from build123d import *

# Parameters (mm, degrees)
BOSS_EXTRUDE1_DEPTH = 34.5
FILLET1_R           = 1
CUT_EXTRUDE1_DEPTH  = 8
FILLET2_R           = 5
SKETCH3_R           = 1.25
CUT_EXTRUDE2_DEPTH  = 8


with BuildPart() as part:
    # Sketch1 → Boss-Extrude1 (new body, symmetric)
    with BuildSketch(Plane.XY):
        with BuildLine():
            Line((-12, -1), (-2.987055406, -1))
            ThreePointArc((-2.987055406, -1), (0, -3.15), (2.987055406, -1))
            Line((2.987055406, -1), (12, -1))
            Line((12, -1), (12, -8))
            Line((12, -8), (-12, -8))
            Line((-12, -8), (-12, -1))
        make_face()
    extrude(amount=BOSS_EXTRUDE1_DEPTH, both=True)

    # Fillet1
    fillet1_edges = [part.edges().sort_by_distance(p)[0] for p in [
        (-2.987055406, -1, 0),
        (2.987055406, -1, 0),
    ]]
    fillet(fillet1_edges, radius=FILLET1_R)

    # Sketch2 → Cut-Extrude1 (cut, through all)
    with BuildSketch(Plane(origin=(0, -1, 0), x_dir=(1, 0, 0), z_dir=(0, 1, 0))):
        Polygon((-12, 27.5), (-5, 19.686646885), (-5, -19.686646885), (-12, -27.5), align=None)
        Polygon((12, -27.5), (5, -19.686646885), (5, 19.686646885), (12, 27.5), align=None)
    extrude(amount=-CUT_EXTRUDE1_DEPTH, mode=Mode.SUBTRACT)

    # Fillet2
    fillet2_edges = [part.edges().sort_by_distance(p)[0] for p in [
        (-12, -4.5, 27.5),
        (-12, -4.5, -27.5),
        (-5, -4.5, -19.686646885),
        (-5, -4.5, 19.686646885),
        (12, -4.5, -27.5),
        (12, -4.5, 27.5),
        (5, -4.5, 19.686646885),
        (5, -4.5, -19.686646885),
    ]]
    fillet(fillet2_edges, radius=FILLET2_R)

    # Sketch3 → Cut-Extrude2 (cut, through all)
    with BuildSketch(Plane(origin=(0, -1, 0), x_dir=(1, 0, 0), z_dir=(0, 1, 0))):
        with Locations((5.25, 29.610191819)):
            Circle(SKETCH3_R)
        with Locations((-5.25, 29.610191819)):
            Circle(SKETCH3_R)
        with Locations((-5.25, -29.610191819)):
            Circle(SKETCH3_R)
        with Locations((5.25, -29.610191819)):
            Circle(SKETCH3_R)
    extrude(amount=-CUT_EXTRUDE2_DEPTH, mode=Mode.SUBTRACT)


solid = part.part
Design review of the part built by this model. Coordinates are the model's own, in mm. A direction names the side the tool comes from. Coordinates: 2 decimals unless noted, no trailing zeros. Order: outer loops, then holes, each group sorted by start corner. A loop starts at its lowest first (then second) coordinate and runs counter-clockwise, first axis right, second up. Notation, with made-up numbers: (60, 84) -> (92, 84) arc R20 cw to (92, 105) -> close; hole circle Ø8 at (-25.5, 22.5). An arc over 180 degrees is marked (long way). One line per item, written item: value.
1) Draft analysis for pull direction X (two halves, no side actions). For faces 4 (the face through (4.98, -4.45, -28.39)), 5 (the face through (-11.66, -4.55, 27.6)), 6 (the face through (5.32, -4.55, 19.54)), state which applies: +X half, -X half, draft (parallel to the pull), parting line (faces both ways), or undercut.
Output values:
face 4: undercut
face 5: -X half
face 6: +X half
2) We need section A-A, the plane z = 8. Give the boundary of the cut face in (x, y).
Output values:
outline: (-5, -8) -> (5, -8) -> (5, -1) -> (3.64, -1) arc R1 ccw to (2.76, -1.52) arc R3.15 cw to (-2.76, -1.52) arc R1 ccw to (-3.64, -1) -> (-5, -1) -> close
3) Clearance check with flat-ended pins moving along their axes: P1, Ø3, axis at y = -3, z = -19, coming from the -X side; P2, Ø4, axis at x = 0.5, z = -5.5, coming from the +Y side. State where each tip first meets the part, or that it passes through.
Output values:
P1: stops at x = -5.81
P2: stops at y = -1.92
4) Machinability: for faces 1 (the face through (12, -4, 32)), 2 (the face through (-11.68, -4.55, -27.65)), 3 (the face through (11.68, -4.55, -27.65)), which of the approach directions +Z, -Z, +X, -X, +Y, -Y give a long, thin tool a straight path to every point of the face, cutting with its end or side? Answer none if there is none.
Output values:
face 1: +Z, -Z, +X, +Y, -Y
face 2: -X, +Y, -Y
face 3: +X, +Y, -Y
5) To check wall thickness, follow probe 1 along Z at (x, y) = (-5.5, -3.5); probe 2 along X at (y, z) = (-7.25, -11.5); probe 3 along Z at (x, y) = (10.5, -3.5). State the ranges of each line that lie inside material, in increasing order. Write a range as [from, to].
Output values:
probe 1: z = [-34.5, -30.83], [-28.39, -19.95], [19.95, 28.39], [30.83, 34.5]
probe 2: x = [-5, 5]
probe 3: z = [-34.5, -25.83], [25.83, 34.5]
6) We need section B-B, the plane x = 8.5. Give the boundary of the cut face in (y, z), then the cut area to 3 significant figures.
Output values:
outline: (-8, -34.5) -> (-1, -34.5) -> (-1, -23.59) -> (-8, -23.59) -> close; (-8, 23.59) -> (-1, 23.59) -> (-1, 34.5) -> (-8, 34.5) -> close
area: 153 mm2
7) We need section D-D, the plane y = -5.5. Give the boundary of the cut face in (x, z), then the cut area to 3 significant figures.
Output values:
outline: (-12, -34.5) -> (12, -34.5) -> (12, -29.41) arc R5 ccw to (10.72, -26.08) -> (6.28, -21.11) arc R5 cw to (5, -17.77) -> (5, 17.77) arc R5 cw to (6.28, 21.11) -> (10.72, 26.08) arc R5 ccw to (12, 29.41) -> (12, 34.5) -> (-12, 34.5) -> (-12, 29.41) arc R5 ccw to (-10.72, 26.08) -> (-6.28, 21.11) arc R5 cw to (-5, 17.77) -> (-5, -17.77) arc R5 cw to (-6.28, -21.11) -> (-10.72, -26.08) arc R5 ccw to (-12, -29.41) -> close; hole circle Ø2.5 at (-5.25, -29.61); hole circle Ø2.5 at (-5.25, 29.61); hole circle Ø2.5 at (5.25, -29.61); hole circle Ø2.5 at (5.25, 29.61)
area: 976 mm2
8) We need section C-C, the plane y = -2.5. Give the boundary of the cut face in (x, z), then the cut area to 3 significant figures.
Output values:
outline: (-12, -34.5) -> (-1.92, -34.5) -> (-1.92, 34.5) -> (-12, 34.5) -> (-12, 29.41) arc R5 ccw to (-10.72, 26.08) -> (-6.28, 21.11) arc R5 cw to (-5, 17.77) -> (-5, -17.77) arc R5 cw to (-6.28, -21.11) -> (-10.72, -26.08) arc R5 ccw to (-12, -29.41) -> close; (1.92, -34.5) -> (12, -34.5) -> (12, -29.41) arc R5 ccw to (10.72, -26.08) -> (6.28, -21.11) arc R5 cw to (5, -17.77) -> (5, 17.77) arc R5 cw to (6.28, 21.11) -> (10.72, 26.08) arc R5 ccw to (12, 29.41) -> (12, 34.5) -> (1.92, 34.5) -> close; hole circle Ø2.5 at (-5.25, -29.61); hole circle Ø2.5 at (-5.25, 29.61); hole circle Ø2.5 at (5.25, -29.61); hole circle Ø2.5 at (5.25, 29.61)
area: 711 mm2
